Part print with two shaded views. Sizes in mm from the minimum x, y, z corner. Give positions to 0.01 mm unless a question says otherwise; leave off trailing zeros. Order: outer loops, then holes, each group sorted by start corner. A loop starts at its lowest first (then second) coordinate and runs counter-clockwise, first axis right, second up. Notation, with made-up numbers: M 39.25,50 L 91.25,50 A26 ccw 91.25,79 Z; hole C 65.25,19.5 d8. An arc over 180 degrees is marked long. Answer as CSV lines item,"result".
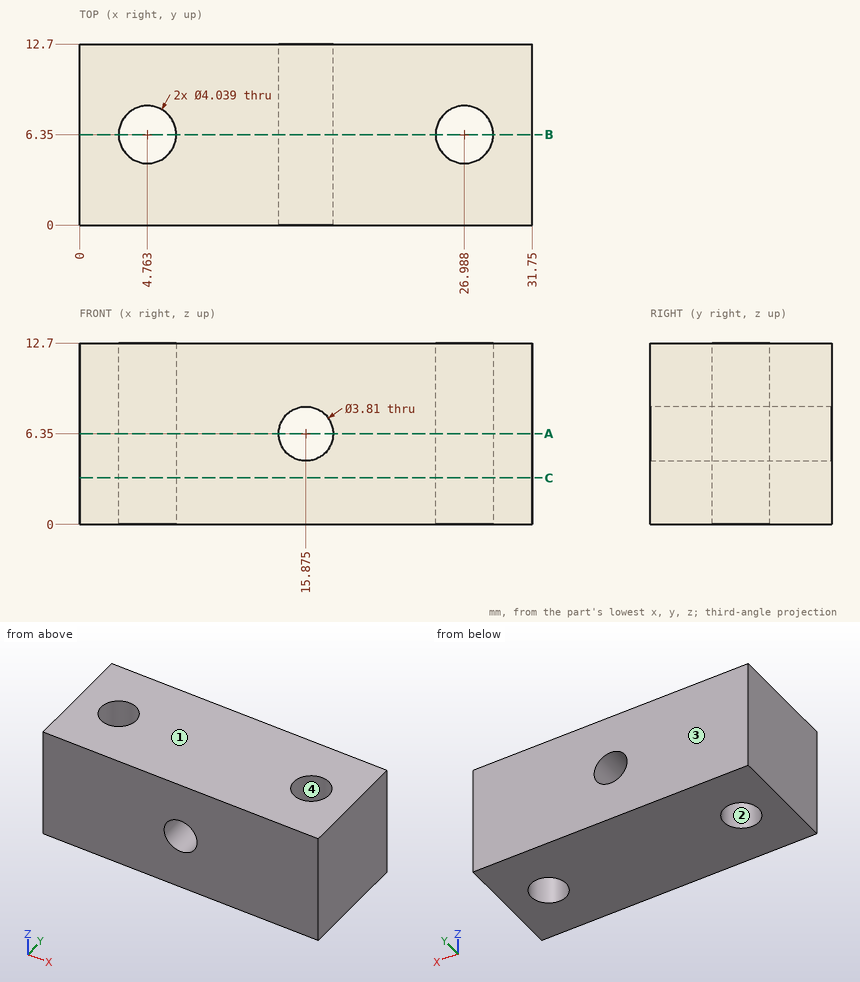
Item 1: Drop a flat-ended pin along its axis: pin 1 (3 mm diameter, centred on x = 26.99, y = 6.35, fed in from +Z). Give the stop position or say it passes through.
Geometry says:
pin 1,"passes through"
Item 2: Band-saw the part on B-B (y = 6.35). State how many separate pieces and enclosed holes the cut face has, and give its area (3 significant figures).
Geometry says:
separate pieces,"3"
enclosed holes,"1"
area,"289 mm2"
Item 3: Band-saw the part on C-C (z = 3.25). Give the cut face in (x, y).
Geometry says:
outline,"M 0,0 L 31.75,0 L 31.75,12.7 L 0,12.7 Z; hole C 4.76,6.35 d4.04; hole C 26.99,6.35 d4.04"
Item 4: Pull direction Y, two halves, no side cores. Call the marked faces 1, 2, 3 and 4: released by +Y, released by -Y, zero draft, split by the parting line, or undercut.
Geometry says:
face 1,"zero draft"
face 2,"undercut"
face 3,"released by +Y"
face 4,"undercut"
Item 5: Band-saw the part on A-A (z = 6.35). Give the cut face in (x, y).
Geometry says:
outline,"M 0,0 L 13.97,0 L 13.97,12.7 L 0,12.7 Z; M 17.78,0 L 31.75,0 L 31.75,12.7 L 17.78,12.7 Z; hole C 4.76,6.35 d4.04; hole C 26.99,6.35 d4.04"
Item 6: Probe line 1 along Y through (x, z) = (27, 12); line 2 along X through (y, z) = (9.5, 6.35); line 3 along Y through (x, z) = (26, 1). List the from-to ranges inside material, lowest first. Write a range as from..to.
Geometry says:
line 1,"y = 0..4.33, 8.37..12.7"
line 2,"x = 0..13.97, 17.78..31.75"
line 3,"y = 0..4.59, 8.11..12.7"
